from build123d import *

# Parameters (mm, degrees)
BOSS_EXTRUDE1_DEPTH = 3
FILLET2_R           = 5
SKETCH2_R           = 6.5
SKETCH2_R_2         = 2.6
SKETCH2_R_3         = 1.6
CUT_EXTRUDE1_DEPTH  = 4.0000001


with BuildPart() as part:
    # Sketch1 → Boss-Extrude1 (new body)
    with BuildSketch(Plane(origin=(0, 0, 0), x_dir=(0, 0, -1), z_dir=(1, 0, 0))):
        with BuildLine():
            ThreePointArc((-41.386624325, 0), (-33.610207892, 10.053296954), (-21.925290889, 5.052882289))
            ThreePointArc((-21.925290889, 5.052882289), (14.009999081, -17.60596279), (0, 22.5))
            Line((0, 22.5), (-32.886624325, 22.5))
            ThreePointArc((-32.886624325, 22.5), (-48.850275915, 17.272163951), (-58.62909831, 3.614086692))
            ThreePointArc((-58.62909831, 3.614086692), (-52.232936073, -8.808582913), (-41.386624325, 0))
        make_face()
    extrude(amount=BOSS_EXTRUDE1_DEPTH)

    # Fillet2
    fillet2_edges = [part.edges().sort_by_distance(p)[0] for p in [
        (1.5, 5.052882289, 21.925290889),
    ]]
    fillet(fillet2_edges, radius=FILLET2_R)

    # Sketch2 → Cut-Extrude1 (cut, through all)
    with BuildSketch(Plane(origin=(3, 0, 0), x_dir=(0, 0, -1), z_dir=(1, 0, 0))):
        Circle(SKETCH2_R)
        with Locations((-50.386624325, 0)):
            Circle(SKETCH2_R_2)
        with Locations((0, 17)):
            Circle(SKETCH2_R_3)
        with Locations((14.722431864, 8.5)):
            Circle(SKETCH2_R_3)
        with Locations((14.722431864, -8.5)):
            Circle(SKETCH2_R_3)
        with Locations((0, -17)):
            Circle(SKETCH2_R_3)
        with Locations((-14.722431864, -8.5)):
            Circle(SKETCH2_R_3)
        with Locations((-14.722431864, 8.5)):
            Circle(SKETCH2_R_3)
    extrude(amount=-CUT_EXTRUDE1_DEPTH, mode=Mode.SUBTRACT)


solid = part.part
Input: part model. Units: mm. Frame: model coordinates. Give positions to 0.01 mm unless a question says otherwise; leave off trailing zeros. Loops run counter-clockwise (first coordinate to the right, second up) from the corner with the lowest first, then second, coordinate; pieces in that order, holes last. Notation, with made-up numbers: (71, -12) -> (83, -12) arc R21 ccw to (83, 0) -> close; hole circle Ø3 at (61.25, 48.5). An arc over 180 degrees is marked (long way). Answer as a JSON object with one key per item and string values. Group by question number.
Item 1: Cut plane B-B, the plane y = -17. Return the cut outline in (x, z).
Item 2: Pull-direction query (Z, two-part tool) for faces 1 (the cylindrical face through (1.521, 7.887, 13.244)), 2 (the cylindrical face through (1.521, -9.113, 13.244)), 3 (the cylindrical face through (1.48, 17.41, 48.66)), 4 (the flat face through (3, 5, 10)); classes: released by +Z, released by -Z, zero draft, split by the parting line, or undercut.
Item 3: Pin query (flat end, axial travel): P1, Ø1, axis at x = 2.5, z = 36.5, coming from the +Y side. Return the tip coordinate at first contact, or that it passes through.
Item 4: Cut plane C-C, the plane z = -2.5. Return the cut outline in (x, y).
Item 5: Line query: probe 1 along Z at (x, y) = (0.9, -8); probe 2 along Z at (x, y) = (2.35, 8); probe 3 along Z at (x, y) = (0.8, 3.5). Output: solid intervals per line, ascending.
Item 6: Cut plane D-D, the plane x = 1.5. State how many separate pieces and enclosed holes the cut face has, and give its area (3 significant figures).
Item 7: Cut plane A-A, the plane z = -14. Return the cut outline in (x, y).
Checks:
{
 "1": {"outline": "(0, -14.74) -> (3, -14.74) -> (3, -1.6) -> (0, -1.6) -> close; (0, 1.6) -> (3, 1.6) -> (3, 14.74) -> (0, 14.74) -> close"},
 "2": {"face 1": "undercut", "face 2": "undercut", "face 3": "released by +Z", "face 4": "zero draft"},
 "3": {"P1": "stops at y = 22.32"},
 "4": {"outline": "(0, -22.36) -> (3, -22.36) -> (3, -6) -> (0, -6) -> close; (0, 6) -> (3, 6) -> (3, 22.36) -> (0, 22.36) -> close"},
 "5": {"probe 1": "z = -21.03 to -16.24, -13.2 to 13.2, 16.24 to 21.03, 46.26 to 54.51", "probe 2": "z = -21.03 to -16.24, -13.2 to 13.2, 16.24 to 24.38, 37.62 to 56.81", "probe 3": "z = -22.23 to -5.48, 5.48 to 22.24, 40.78 to 58.68"},
 "6": {"separate pieces": "1", "enclosed holes": "8", "area": "2,150 mm²"},
 "7": {"outline": "(0, -17.61) -> (3, -17.61) -> (3, -9.93) -> (0, -9.93) -> close; (0, -7.07) -> (3, -7.07) -> (3, 7.07) -> (0, 7.07) -> close; (0, 9.93) -> (3, 9.93) -> (3, 17.61) -> (0, 17.61) -> close"}
}
